Geometry: final body of the model. Coordinates: model frame, mm. Face numbers are marked on the shaded views. Coordinates: 2 decimals unless noted, no trailing zeros. Loops run counter-clockwise (first coordinate to the right, second up) from the corner with the lowest first, then second, coordinate; pieces in that order, holes last. Notation, with made-up numbers: (70.5, -8.5) - (94.5, -8.5) arc R12 cw to (94.5, 6.5) - close; hole circle Ø3 at (70, 36). An arc over 180 degrees is marked (long way). Put each result on its own line as item: value. Start each with the question number.
1) Contact query for flat-ended pins moving along their axis: pin 1 Ø1.5 at (x, z) = (28, 15.5) entering from +Y; pin 2 Ø5 at (x, z) = (32.5, -9.5) entering from -Y; pin 3 Ø23 at (x, z) = (0, 0) entering from +Y. Output: stop coordinate, or through.
2) Section D-D on y = 15. Output: boundary loops of the cut face in (x, z).
3) Draft query along Z for the marked faces 1, 2 and 3. Return one class per face: +Z half, -Z half, draft (parallel to the pull), parting line (faces both ways), or undercut.
4) Section B-B on x = 30. Output: boundary loops of the cut face in (y, z).
5) Material intervals for line 1 along Y through (x, z) = (34.75, 0); line 2 along X through (y, z) = (18.5, 15.5); line 3 along X through (y, z) = (14.5, 2), sorted ascending. Write a range as from..to.
6) Section A-A on z = 0. Output: boundary loops of the cut face in (x, y).
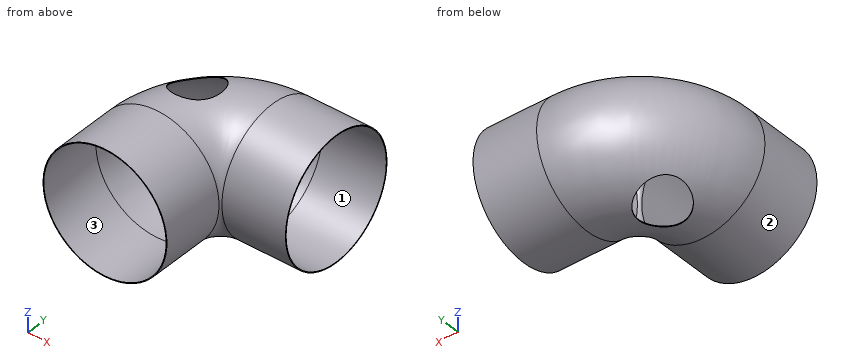
Autodesk Inventor part; units mm, degrees
ref_plane "YZ Plane" through (0, 0, 0) normal (1, 0, 0) x (0, 1, 0)
ref_plane "XZ Plane" through (0, 0, 0) normal (0, 1, 0) x (-1, 0, 0)
ref_plane "XY Plane" through (0, 0, 0) normal (0, 0, 1) x (1, 0, 0)
sketch "Sketch1" plane through (0, 0, 0) normal (0, 0, 1) x (1, 0, 0)
  line L0 (0, 0) -> (0, 20)
  line L1 (20, 40) -> (40, 40)
  arc A0 (20, 40) -> (0, 20) centre (20, 20) ccw
  point P0 (0, 40)
  dimension "d0" = 40
  dimension "d1" = 40
  dimension "d2" = 20
sketch "Sketch2" plane through (0, 0, 0) normal (0, 1, 0) x (-1, 0, 0)
  circle A0 centre (0, 0) radius 19.5
  circle A1 centre (0, 0) radius 19.25
  dimension "d3" = 39
  dimension "d4" = 38.5
sweep "Sweep1" add profiles "Sketch2" path "Sketch1"
sketch "Sketch4" plane through (0, 0, 0) normal (0, 0, 1) x (1, 0, 0)
  circle A0 centre (0, 35.5061) radius 7.5
  point P0 (0, 0)
  dimension "d10" = 15
extrude "Extrusion2" cut sketch "Sketch4" against normal mid plane 40
properties part number "elb"
Answer block:
1. pin 1: stops at y = 52.75
1. pin 2: stops at y = 21.8
1. pin 3: stops at y = 58.57
2. outline: circle Ø39 at (0, 0); hole circle Ø38.5 at (0, 0)
3. face 1: undercut
3. face 2: parting line
3. face 3: undercut
4. outline: circle Ø39 at (40, 0); hole circle Ø38.5 at (40, 0)
5. line 1: y = 20.5..20.75, 59.25..59.5
5. line 2: x = -11.83..-11.42, 11.42..11.83
5. line 3: x = -19.4..-19.15, 19.15..19.4
6. outline: (-19.5, 0) - (-19.25, 0) - (-19.25, 20) arc R39.25 cw to (20, 59.25) - (40, 59.25) - (40, 59.5) - (20, 59.5) arc R39.5 ccw to (-19.5, 20) - close; (19.25, 0) - (19.5, 0) - (19.5, 20) arc R0.5 cw to (20, 20.5) - (40, 20.5) - (40, 20.75) - (20, 20.75) arc R0.75 ccw to (19.25, 20) - close
